The listing builds one solid part. Answer for the finished solid, in the listing's coordinates (mm). A direction names the side the tool comes from. Give positions to 0.01 mm unless a question says otherwise; leave off trailing zeros. Write each loop counter-clockwise with the first axis right and the second up, starting at its lowest first coordinate (ties: lowest second). Pieces come first, ordered by that corner, then holes. Notation, with made-up numbers: (51.5, -11) -> (74.5, -11) arc R31 cw to (74.5, 19) -> close; hole circle Ø2 at (85, -8.75). An arc over 180 degrees is marked (long way). Use CSV: the item, a comma, the result in double quotes. Start each with the question number.
from build123d import *

# Parameters (mm, degrees)
SKETCH1_W                                           = 354
SKETCH1_H                                           = 16
BOSS_EXTRUDE1_DEPTH                                 = 15
M5_TAPPED_HOLE1_D                                   = 4.2
SKETCH7_W                                           = 25
SKETCH7_H                                           = 27.047818694
CUT_EXTRUDE2_DEPTH                                  = 179.353581405
CHAMFER1_SIZE                                       = 2
CHAMFER1_OF_MIRROR1_SIZE                            = 2
G1_8_TAPPED_HOLE1_D                                 = 8.8
G1_8_TAPPED_HOLE1_DEPTH                             = 9
G1_8_TAPPED_HOLE1_TIP                               = 2.643786724
SKETCH10_W                                          = 30
SKETCH10_H                                          = 18
CUT_EXTRUDE3_DEPTH                                  = 179.353581405
CBORE_FOR_M6_HEX_SOCKET_HEAD_CAP_SCREW1_D           = 6.6
CBORE_FOR_M6_HEX_SOCKET_HEAD_CAP_SCREW1_CBORE_D     = 11
CBORE_FOR_M6_HEX_SOCKET_HEAD_CAP_SCREW1_CBORE_DEPTH = 6.4


with BuildPart() as part:
    # Sketch1 → Boss-Extrude1 (new, symmetric)
    with BuildSketch(Plane(origin=(0, 0, 0), x_dir=(1, 0, 0), z_dir=(0, 1, 0))):
        Rectangle(SKETCH1_W, SKETCH1_H)
    extrude(amount=BOSS_EXTRUDE1_DEPTH, both=True)

    # M5 Tapped Hole1 (through all)
    with Locations(Plane(origin=(0, 15, 0), x_dir=(1, 0, 0), z_dir=(0, 1, 0))):
        with Locations((-110, 0), (110, 0)):
            Hole(M5_TAPPED_HOLE1_D / 2)

    # Sketch7 → Cut-Extrude2 (cut, through all)
    with BuildSketch(Plane.XY.offset(8)):
        with Locations((110, -13.023909347)):
            Rectangle(SKETCH7_W, SKETCH7_H)
    cut_extrude2 = extrude(amount=-CUT_EXTRUDE2_DEPTH, mode=Mode.SUBTRACT)

    # Chamfer1
    chamfer1_edges = [part.edges().sort_by_distance(p)[0] for p in [
        (122.5, -15, 0),
        (97.5, -15, 0),
    ]]
    chamfer(chamfer1_edges, length=CHAMFER1_SIZE)

    # Mirror1: Cut-Extrude2 across plane
    add(cut_extrude2.mirror(Plane(origin=(0, 0, 0), x_dir=(0, 0, 1), z_dir=(1, 0, 0))), mode=Mode.SUBTRACT)

    # Chamfer1 of Mirror1
    chamfer1_of_mirror1_edges = [part.edges().sort_by_distance(p)[0] for p in [
        (-122.5, -15, 0),
        (-97.5, -15, 0),
    ]]
    chamfer(chamfer1_of_mirror1_edges, length=CHAMFER1_OF_MIRROR1_SIZE)

    # G1/8 Tapped Hole1
    with Locations(Plane(origin=(0, 15, 0), x_dir=(1, 0, 0), z_dir=(0, 1, 0))):
        with Locations((-110, 0), (110, 0)):
            Hole(G1_8_TAPPED_HOLE1_D / 2, depth=G1_8_TAPPED_HOLE1_DEPTH)
            with Locations((0, 0, -(G1_8_TAPPED_HOLE1_DEPTH + G1_8_TAPPED_HOLE1_TIP / 2))):  # 118° drill point
                Cone(0, G1_8_TAPPED_HOLE1_D / 2, G1_8_TAPPED_HOLE1_TIP, mode=Mode.SUBTRACT)

    # Sketch10 → Cut-Extrude3 (cut, through all)
    with BuildSketch(Plane.XY.offset(8)):
        with Locations((-162, 6)):
            Rectangle(SKETCH10_W, SKETCH10_H)
    cut_extrude3 = extrude(amount=-CUT_EXTRUDE3_DEPTH, mode=Mode.SUBTRACT)

    # Mirror2: Cut-Extrude3 across plane
    add(cut_extrude3.mirror(Plane(origin=(0, 0, 0), x_dir=(0, 0, 1), z_dir=(1, 0, 0))), mode=Mode.SUBTRACT)

    # CBORE for M6 Hex Socket Head Cap Screw1 (through all)
    with Locations(Plane(origin=(0, -15, 0), x_dir=(-1, 0, 0), z_dir=(0, -1, 0))):
        with Locations((-160, 0), (160, 0)):
            CounterBoreHole(CBORE_FOR_M6_HEX_SOCKET_HEAD_CAP_SCREW1_D / 2, CBORE_FOR_M6_HEX_SOCKET_HEAD_CAP_SCREW1_CBORE_D / 2, CBORE_FOR_M6_HEX_SOCKET_HEAD_CAP_SCREW1_CBORE_DEPTH)


solid = part.part
Q1. For faces 1 (the face through (166, -3, 0)), 2 (the face through (113, 0.5, 0)), 3 (the face through (-105.604, 10.437, -0.193)), 4 (the face through (-160, -8.6, 4)), 5 (the face through (-2, 15, 0)), determine the directions among +Z, -Z, +X, -X, +Y, -Y from which every point of the face is accessible in a straight line to the end or side of a thin tool.
Q2. The mould has two halves that part along Z. Classify faces 6 (the face through (-147, 6, 0)), 7 (the face through (165.495, -11.845, -0.242)): +Z half, -Z half, draft (parallel to the pull), parting line (faces both ways), or undercut.
Q3. Section A-A on x = -160 is taken. Give the vertices of the cut face in (y, z).
Q4. Section B-B on y = 9 is taken. Give the vertices of the cut face in (x, z), then the cut area to 3 significant figures.
Q5. Flat-ended cylindrical pins translate along their axes: pin 1 Ø7.5 at (x, z) = (-160, 0) entering from +Y; pin 2 Ø1.5 at (y, z) = (-2, -1) entering from -X; pin 3 Ø8 at (y, z) = (9, 4) entering from +X. Find the tip coordinate at first contact, or state that the pin passes through.
Q6. Straight lines are drawn through the part: L1, parallel to X at y = 7.5, z = -0.25; L2, parallel to Z at x = 110, y = 1.45; L3, parallel to Z at x = -160, y = -11.5. For each, find the intervals that lie inside material, in ascending order.
Output:
1,face 1,"+Z, -Z, +X, +Y"
1,face 2,"+Z, -Z, -Y"
1,face 3,"+Y"
1,face 4,"-Y"
1,face 5,"+Z, -Z, +X, -X, +Y"
2,face 6,"draft"
2,face 7,"undercut"
3,outline,"(-15, -8) -> (-3, -8) -> (-3, -3.3) -> (-8.6, -3.3) -> (-8.6, -5.5) -> (-15, -5.5) -> close; (-15, 5.5) -> (-8.6, 5.5) -> (-8.6, 3.3) -> (-3, 3.3) -> (-3, 8) -> (-15, 8) -> close"
4,outline,"(-147, -8) -> (147, -8) -> (147, 8) -> (-147, 8) -> close; hole circle Ø8.8 at (-110, 0); hole circle Ø8.8 at (110, 0)"
4,area,"4,580 mm²"
5,pin 1,"y = -3"
5,pin 2,"x = -147"
5,pin 3,"x = 147"
6,L1,"-147 to -114.39, -105.61 to 105.61, 114.39 to 147"
6,L2,"-8 to -2.1, 2.1 to 8"
6,L3,"-8 to -5.5, 5.5 to 8"
